Autodesk Inventor part; units mm, degrees
ref_plane "YZ Plane" through (0, 0, 0) normal (1, 0, 0) x (0, 1, 0)
ref_plane "XZ Plane" through (0, 0, 0) normal (0, 1, 0) x (-1, 0, 0)
ref_plane "XY Plane" through (0, 0, 0) normal (0, 0, 1) x (1, 0, 0)
sketch "Sketch1" plane through (0, 0, 0) normal (0, 0, 1) x (1, 0, 0)
  line L0 (-10, -10) -> (10, -10)
  line L1 (10, -10) -> (10, 10)
  line L2 (10, 10) -> (-10, 10)
  line L3 (-10, 10) -> (-10, -10)
  line L4 (-10, -10) -> (10, 10) construction
  line L5 (10, -10) -> (-10, 10) construction
  circle A0 centre (0, 0) radius 2.4
  dimension "d0" = 20
  dimension "d1" = 20
  dimension "d2" = 4.8
extrude "Extrusion1" add sketch "Sketch1" along normal blind 2
chamfer "Chamfer1" distance 0.5 angle 45 4 edges at (10, 0, 0) (0, 10, 0) (-10, 0, 0) (0, -10, 0)
sketch "Sketch2" plane through (0, 0, 2) normal (0, 0, 1) x (1, 0, 0)
  line L0 (10, 10) -> (10, -10)
  line L1 (-10, -6) -> (10, -6)
  line L2 (10, -6) -> (10, 6)
  line L3 (10, 6) -> (-10, 6)
  line L4 (-10, 6) -> (-10, -6)
  line L5 (-10, -6) -> (10, 6) construction
  line L6 (10, -6) -> (-10, 6) construction
  point P0 (0, 0)
  point P1 (10, -6)
  dimension "d8" = 12
extrude "Extrusion2" add sketch "Sketch2" along normal blind 5
sketch "Sketch5" plane through (-10, -6, 2) normal (0, -1, 0) x (1, 0, 0)
  line L0 (20, 0) -> (0, 0)
  line L1 (3, 0) -> (17, 0)
  line L2 (17, 0) -> (17, 3)
  line L3 (17, 3) -> (3, 3)
  line L4 (3, 3) -> (3, 0)
  line L5 (0, 0) -> (0, 5)
  line L6 (20, 0) -> (20, 5)
  point P0 (10, -2)
  dimension "d18" = 3
  dimension "d19" = 3
  dimension "d20" = 3
extrude "Extrusion4" cut sketch "Sketch5" against normal through all
sketch "Sketch6" plane through (0, 0, 7) normal (0, 0, 1) x (1, 0, 0)
  circle A0 centre (0, 0) radius 2.4 construction
  circle A1 centre (0, 0) radius 4
  dimension "d23" = 8
extrude "Extrusion5" cut sketch "Sketch6" against normal up to surface (5 mm away)
chamfer "Chamfer4" distance 1.5 angle 45 2 edges at (-7, 0, 5) (7, 0, 5)
chamfer "Chamfer5" distance 1.5 angle 45 6 edges at (0, -6, 5) (0, 6, 5) (-6.25, -6, 4.25) (6.25, -6, 4.25) (6.25, 6, 4.25) (-6.25, 6, 4.25)
chamfer "Chamfer6" distance 1.5 angle 45 2 edges at (-10, 0, 7) (10, 0, 7)
chamfer "Chamfer7" distance 2 angle 45 8 edges at (10, 10, 1.25) (-10, 10, 1.25) (-10, -10, 1.25) (10, -10, 1.25) (8.5, -6, 2) (-8.5, -6, 2) (-8.5, 6, 2) (8.5, 6, 2)
properties part number "CableHolder"
Source: CAD feature listing. Evaluate the final solid. Frame: model axes, mm. A direction names the side the tool comes from. Round coordinates to 2 decimals unless told otherwise and drop trailing zeros. Loops run counter-clockwise (first coordinate to the right, second up) from the corner with the lowest first, then second, coordinate; pieces in that order, holes last. Notation, with made-up numbers: (9.5, 88.25) -> (14.5, 88.25) arc R29 ccw to (14.5, 118.25) -> close; hole circle Ø4 at (42, -19.5). An arc over 180 degrees is marked (long way). Answer as a JSON object with one key per item and string values. Group by question number.
Q1. Contact query for flat-ended pins moving along their axis: P1, Ø0.9, axis at x = -0.5, z = 5, coming from the -Y side; P2, Ø0.9, axis at x = -4, z = 5.5, coming from the +Y side. Output: stop coordinate, or through.
Q2. Section query A-A (y = 0). Output: boundary loops of the cut face in (x, z).
Q3. Section query B-B (z = 1). Output: boundary loops of the cut face in (x, y), plus the area to 3 significant figures.
Q4. Section query D-D (z = 3). Output: boundary loops of the cut face in (x, y).
Q5. Section query C-C (x = 5.25). Output: boundary loops of the cut face in (y, z).
Q6. Ray query, line 1 (Z direction, x = -6.5, y = 3.25); line 2 (Y direction, x = 0, z = 6.65); line 3 (Y direction, x = 0, z = 1.25). Return the intervals inside material, ascending. Write a range as from..to.
Q7. Mould query, pull axis X, two halves, no side actions, for faces 1 (the flat face through (-2, 2, 0)), 2 (the flat face through (-6.351, 5.239, 5.194)), 3 (the flat face through (-9, -9, 1)). Classes: pulls with the +X half, pulls with the -X half, needs draft (parallel to the pull), parting line crosses it, or undercut.
Q8. Access query for faces 4 (the flat face through (6.54, 5.24, 5.01)), 5 (the flat face through (-0.1, -5.3, 5.8)), 6 (the flat face through (-6.3, -0.1, 4.2)). Directions: +Z, -Z, +X, -X, +Y, -Y. A direction counts if a zero-diameter tool reaches every point of the face in a straight line with its end or side. Return the directions, or none.
Completed:
{
 "1": {"P1": "y = -4.95", "P2": "y = 5.45"},
 "2": {"outline": "(-10, 0.5) -> (-9.5, 0) -> (-2.4, 0) -> (-2.4, 2) -> (-7, 2) -> (-7, 3.5) -> (-5.5, 5) -> (-4, 5) -> (-4, 7) -> (-8.5, 7) -> (-10, 5.5) -> close; (2.4, 0) -> (9.5, 0) -> (10, 0.5) -> (10, 5.5) -> (8.5, 7) -> (4, 7) -> (4, 5) -> (5.5, 5) -> (7, 3.5) -> (7, 2) -> (2.4, 2) -> close"},
 "3": {"outline": "(-10, -8) -> (-8, -10) -> (8, -10) -> (10, -8) -> (10, 8) -> (8, 10) -> (-8, 10) -> (-10, 8) -> close; hole circle Ø4.8 at (0, 0)", "area": "374 mm²"},
 "4": {"outline": "(-10, -7) -> (-7, -7) -> (-7, 7) -> (-10, 7) -> close; (7, -7) -> (10, -7) -> (10, 7) -> (7, 7) -> close"},
 "5": {"outline": "(-10, 0.5) -> (-9.5, 0) -> (9.5, 0) -> (10, 0.5) -> (10, 2) -> (-10, 2) -> close; (-6, 6.5) -> (-4.5, 5) -> (4.5, 5) -> (6, 6.5) -> (6, 7) -> (-6, 7) -> close"},
 "6": {"line 1": "0..2, 4..7", "line 2": "-6..-4, 4..6", "line 3": "-10..-2.4, 2.4..10"},
 "7": {"face 1": "needs draft", "face 2": "undercut", "face 3": "pulls with the -X half"},
 "8": {"face 4": "+Y", "face 5": "-Y", "face 6": "+Y, -Y"}
}
